```python
from build123d import *

# Parameters (mm, degrees)
SKETCH_1_R                 = 32
EXTRUDE_1_DEPTH            = 20.5
SKETCH_12_R                = 45
EXTRUDE_2_DEPTH            = 15
SKETCH_11_R                = 29
CUT_EXTRUDE_6_DEPTH        = 35.5
SKETCH_13_R                = 42
CUT_EXTRUDE_7_DEPTH        = 11
HOLE_START                 = 20.5
HOLE_WIZARD_M3_1_OUTLINE_R = 1.25
HOLE_WIZARD_M3_1_DEPTH     = 4


# Read off the part's stored shape, not the designer's step: M3 螺纹孔1
with BuildPart() as part:
    # 草图1 → 凸台-拉伸1 (new body)
    with BuildSketch(Plane(origin=(0, 0, 0), x_dir=(1, 0, 0), z_dir=(0, 1, 0))):
        with Locations(Location((0, 0, 0), (0, 0, 270))):
            Circle(SKETCH_1_R)
    extrude(amount=EXTRUDE_1_DEPTH)

    # 草图12 → 凸台-拉伸2 (add)
    with BuildSketch(Plane(origin=(0, 20.5, 0), x_dir=(1, 0, 0), z_dir=(0, 1, 0))):
        with Locations(Location((0, 0, 0), (0, 0, 270))):
            Circle(SKETCH_12_R)
    extrude(amount=EXTRUDE_2_DEPTH)

    # 草图11 → 切除-拉伸6 (cut)
    with BuildSketch(Plane(origin=(0, 0, 0), x_dir=(1, 0, 0), z_dir=(0, 1, 0))):
        with Locations(Location((0, 0, 0), (0, 0, 90))):
            Circle(SKETCH_11_R)
    extrude(amount=CUT_EXTRUDE_6_DEPTH, mode=Mode.SUBTRACT)

    # 草图13 → 切除-拉伸7 (cut)
    with BuildSketch(Plane(origin=(0, 35.5, 0), x_dir=(1, 0, 0), z_dir=(0, 1, 0))):
        with Locations(Location((0, 0, 0), (0, 0, 270))):
            Circle(SKETCH_13_R)
    extrude(amount=-CUT_EXTRUDE_7_DEPTH, mode=Mode.SUBTRACT)

    # M3 螺纹孔1 outline → M3 螺纹孔1 (cut)
    with BuildSketch(Plane(origin=(0, 0, 0), x_dir=(1, 0, 0), z_dir=(0, 1, 0)).offset(HOLE_START)):
        with Locations((-22.273863607, -22.273863607)):
            Circle(HOLE_WIZARD_M3_1_OUTLINE_R)
        with Locations((22.273863607, -22.273863607)):
            Circle(HOLE_WIZARD_M3_1_OUTLINE_R)
        with Locations((22.273863607, 22.273863607)):
            Circle(HOLE_WIZARD_M3_1_OUTLINE_R)
        with Locations((-22.273863607, 22.273863607)):
            Circle(HOLE_WIZARD_M3_1_OUTLINE_R)
    extrude(amount=HOLE_WIZARD_M3_1_DEPTH, mode=Mode.SUBTRACT)


solid = part.part
```
Part model, mm, in its own coordinate system. A direction names the side the tool comes from. Round coordinates to 2 decimals unless told otherwise and drop trailing zeros. Loops run counter-clockwise (first coordinate to the right, second up) from the corner with the lowest first, then second, coordinate; pieces in that order, holes last.
1. Drill centre lines: line 1 along X through (y, z) = (13.25, 0); line 2 along Y through (x, z) = (-34.5, 2); line 3 along X through (y, z) = (17.5, -14.5). Where is each one in solid material? Low to high.
Solutions:
line 1: x = -32 to -29, 29 to 32
line 2: y = 20.5 to 24.5
line 3: x = -28.53 to -25.11, 25.11 to 28.53
2. Flat gauge pins, fed straight in: pin 1 (1.5 mm diameter, centred on x = 22.27, z = 22.27, fed in from +Y); pin 2 (8 mm diameter, centred on y = 6, z = 24.5, fed in from -X); pin 3 (10 mm diameter, centred on x = -10.5, z = -33.5, fed in from +Y). Where does each tip first touch, or does it go through?
Solutions:
pin 1: stops at y = 20.5
pin 2: stops at x = -24.57
pin 3: stops at y = 24.5
3. 3-axis set-ups, long thin cutter, end or side, ignore diameter. For faces 1 (the face through (-23.195, 22.472, -23.119)), 2 (the face through (-17.235, 27.895, 41.569)), 3 (the face through (31, 20.5, 9)): which of +Z, -Z, +X, -X, +Y, -Y reach the whole face in a straight line?
Solutions:
face 1: +Y
face 2: +Y, -Y
face 3: -Y
4. Slice it at C-C (y = 5.5). Give the cut face in (x, z), and give its area (3 significant figures).
Solutions:
outline: circle Ø64 at (0, 0); hole circle Ø58 at (0, 0)
area: 575 mm2
5. Slice it at B-B (x = 0). Give the cut face in (y, z).
Solutions:
outline: (0, -32) - (20.5, -32) - (20.5, -45) - (35.5, -45) - (35.5, -42) - (24.5, -42) - (24.5, -29) - (0, -29) - close; (0, 29) - (24.5, 29) - (24.5, 42) - (35.5, 42) - (35.5, 45) - (20.5, 45) - (20.5, 32) - (0, 32) - close
6. Two-plate mould, pull along Y, no slides. Class faces 4 (the face through (22, 20.5, -22)), 5 (the face through (29, 0, -5)), 6 (the face through (22.946, 22.472, -23.328)): pulls with the +Y half, pulls with the -Y half, needs draft (parallel to the pull), parting line crosses it, or undercut.
Solutions:
face 4: pulls with the +Y half
face 5: pulls with the -Y half
face 6: needs draft
7. Slice it at D-D (z = -36). Give the cut face in (x, y).
Solutions:
outline: (-27, 20.5) - (27, 20.5) - (27, 35.5) - (21.63, 35.5) - (21.63, 24.5) - (-21.63, 24.5) - (-21.63, 35.5) - (-27, 35.5) - close
8. Slice it at A-A (z = 0). Give the cut face in (x, y), and give its area (3 significant figures).
Solutions:
outline: (-45, 20.5) - (-32, 20.5) - (-32, 0) - (-29, 0) - (-29, 24.5) - (-42, 24.5) - (-42, 35.5) - (-45, 35.5) - close; (29, 0) - (32, 0) - (32, 20.5) - (45, 20.5) - (45, 35.5) - (42, 35.5) - (42, 24.5) - (29, 24.5) - close
area: 317 mm2
